The model under review builds one solid part; all positions refer to its coordinate system, in mm. Coordinates: 2 decimals unless noted, no trailing zeros. Order: outer loops, then holes, each group sorted by start corner. A loop starts at its lowest first (then second) coordinate and runs counter-clockwise, first axis right, second up.
from build123d import *

# Parameters (mm, degrees)
F1_DEPTH = 60
F2_SIZE  = 5
F3_R     = 25
F4_DEPTH = 25
F5_DEPTH = 25
F6_DEPTH = 37.9
F7_SIZE  = 5


with BuildPart() as f1:
    # F0 (on Front) → F1 (new body)
    with BuildSketch(Plane.XZ):
        Polygon((41.7999535799, 43.9688995481), (-58.2000464201, 43.9688995481), (-58.2000464201, -28.3167899087), (-30.4857346934, -56.0311004519), (19.0735861891, -56.0311004519), (41.7999535799, -24.6786684919), align=None)
    extrude(amount=F1_DEPTH)

    # F2
    f2_edges = [f1.edges().sort_by_distance(p)[0] for p in [
        (41.799954, -60, 9.645116),
        (-8.200046, -60, 43.9689),
        (-58.200046, -60, 7.826055),
        (-44.342891, -60, -42.173945),
        (-5.706074, -60, -56.0311),
        (30.43677, -60, -40.354884),
    ]]
    chamfer(f2_edges, length=F2_SIZE)

    # F3 (on Front) → F4 (cut)
    with BuildSketch(Plane.XZ):
        with Locations((-10.7513342236, 0)):
            Circle(F3_R)
    extrude(amount=-F4_DEPTH, mode=Mode.SUBTRACT)

    # F3 (on Front) → F5 (cut)
    with BuildSketch(Plane.XZ):
        with Locations((-10.7513342236, 0)):
            Circle(F3_R)
    extrude(amount=-F5_DEPTH, mode=Mode.SUBTRACT)

    # F3 (on Front) → F6 (cut)
    with BuildSketch(Plane.XZ):
        with Locations((-10.7513342236, 0)):
            Circle(F3_R)
    extrude(amount=F6_DEPTH, mode=Mode.SUBTRACT)

    # F7
    f7_edges = [f1.edges().sort_by_distance(p)[0] for p in [
        (41.799954, 0, 9.645116),
        (30.43677, 0, -40.354884),
        (-8.200046, 0, 43.9689),
        (-5.706074, 0, -56.0311),
        (-58.200046, 0, 7.826055),
        (-44.342891, 0, -42.173945),
        (-35.751334, 0, 0),
    ]]
    chamfer(f7_edges, length=F7_SIZE)


solid = f1.part
(1) Consider section D-D (x = -47). Give the boundary of the cut face in (y, z), then the cut area to 3 significant figures.
(2) The part is to be moulded in two halves that separate along X. For faces 1 (the face through (11, 0, -25)), 2 (the face through (28.225, -57.535, -39.087)), 3 (the face through (-11, -37.9, 0)), say which applies: +X half, -X half, draft (parallel to the pull), parting line (faces both ways), or undercut.
(3) Insertion check: pin 1 Ø4 at (y, z) = (-9, -31.5) entering from +X; pin 2 Ø25 at (x, z) = (-6.5, -7.5) entering from +Y. Each pin has a flat end and moves straight along its axis. Give the tip position at first contact, or say it passes through.
(4) Consider section B-B (z = 0). Give the boundary of the cut face in (x, y).
(5) Consider section C-C (y = -42). Give the boundary of the cut face in (x, z), then the cut area to 3 significant figures.
(6) Wall thickness on line 1 (Y direction, x = -25, z = -20); line 2 (X direction, y = -25, z = 5.5); line 3 (X direction, y = -35.5, z = 9.5): over which ranges is each line inside the solid? List them lowest first.
(7) Consider section A-A (y = -35.5). Give the boundary of the cut face in (x, z), then the cut area to 3 significant figures.
Findings:
1. outline: (-60, -32.45) - (-55, -39.52) - (-5, -39.52) - (0, -32.45) - (0, 38.97) - (-5, 43.97) - (-55, 43.97) - (-60, 38.97) - close
1. area: 4,950 mm2
2. face 1: draft
2. face 2: +X half
2. face 3: undercut
3. pin 1: stops at x = 38.31
3. pin 2: stops at y = -37.9
4. outline: (-58.2, -55) - (-53.2, -60) - (36.8, -60) - (41.8, -55) - (41.8, -5) - (36.8, 0) - (19.25, 0) - (14.25, -5) - (14.25, -37.9) - (-35.75, -37.9) - (-35.75, -5) - (-40.75, 0) - (-53.2, 0) - (-58.2, -5) - close
5. outline: (-58.2, -28.32) - (-30.49, -56.03) - (19.07, -56.03) - (41.8, -24.68) - (41.8, 43.97) - (-58.2, 43.97) - close
5. area: 9,260 mm2
6. line 1: y = -60 to -37.9
6. line 2: x = -58.2 to -35.14, 13.64 to 41.8
6. line 3: x = -58.2 to -33.88, 12.37 to 41.8
7. outline: (-58.2, -28.32) - (-30.49, -56.03) - (19.07, -56.03) - (41.8, -24.68) - (41.8, 43.97) - (-58.2, 43.97) - close; hole circle Ø50 at (-10.75, 0)
7. area: 7,300 mm2
